from build123d import *

# Parameters (mm, degrees)
SKETCH1_R           = 1.8288
BOSS_EXTRUDE1_DEPTH = 3.175
SKETCH2_R           = 1.63195
SKETCH2_R_2         = 5.715
SKETCH2_R_3         = 1.524
CUT_EXTRUDE1_DEPTH  = 4.175
SKETCH3_R           = 1.375
CUT_EXTRUDE2_DEPTH  = 4.175


with BuildPart() as part:
    # Sketch1 → Boss-Extrude1 (new body)
    with BuildSketch(Plane(origin=(0, 0, 0), x_dir=(1, 0, 0), z_dir=(0, 1, 0))):
        Polygon((-226.6315, 82.55), (-194.8815, 82.55), (-194.8815, 69.85), (-188.5315, 69.85), (-188.5315, 82.55), (-38.1, 82.55), (-38.1, 69.85), (-31.75, 69.85), (-31.75, 82.55), (0, 82.55), (0, 51.435), (-3.175, 51.435), (-3.175, 31.115), (0, 31.115), (0, 0), (-31.75, 0), (-31.75, 12.7), (-38.1, 12.7), (-38.1, 0), (-188.5315, 0), (-188.5315, 12.7), (-194.8815, 12.7), (-194.8815, 0), (-226.6315, 0), (-226.6315, 31.115), (-223.4565, 31.115), (-223.4565, 51.435), (-226.6315, 51.435), align=None)
        with Locations((-113.31575, 41.275)):
            Circle(SKETCH1_R, mode=Mode.SUBTRACT)
    extrude(amount=BOSS_EXTRUDE1_DEPTH)

    # Sketch2 → Cut-Extrude1 (cut, through all)
    with BuildSketch(Plane(origin=(0, 3.175, 0), x_dir=(1, 0, 0), z_dir=(0, 1, 0))):
        with Locations((-87.63, 27.305)):
            Circle(SKETCH2_R)
        with Locations((-69.85, 27.305)):
            Circle(SKETCH2_R)
        with Locations((-69.85, 55.245)):
            Circle(SKETCH2_R)
        with Locations((-87.63, 55.245)):
            Circle(SKETCH2_R)
        with Locations((-78.74, 41.275)):
            Circle(SKETCH2_R_2)
        with Locations((-129.82575, 41.275)):
            Circle(SKETCH2_R_3)
        with Locations((-96.80575, 41.275)):
            Circle(SKETCH2_R_3)
    extrude(amount=-CUT_EXTRUDE1_DEPTH, mode=Mode.SUBTRACT)

    # Sketch3 → Cut-Extrude2 (cut, through all)
    with BuildSketch(Plane(origin=(0, 3.175, 0), x_dir=(1, 0, 0), z_dir=(0, 1, 0))):
        with Locations((-174.4315, 57.97)):
            Circle(SKETCH3_R)
        with Locations((-213.9315, 57.97)):
            Circle(SKETCH3_R)
        with Locations((-213.9315, 77.47)):
            Circle(SKETCH3_R)
        with Locations((-174.4315, 77.47)):
            Circle(SKETCH3_R)
    extrude(amount=-CUT_EXTRUDE2_DEPTH, mode=Mode.SUBTRACT)


solid = part.part
Input: part model. Units: mm. Frame: model coordinates. Give positions to 0.01 mm unless a question says otherwise; leave off trailing zeros. Answer as a JSON object with one key per item and string values. Group by question number.
Item 1: Pull-direction query (X, two-part tool) for faces 1 (the cylindrical face through (-113.55, 1.57, -43.09)), 2 (the flat face through (-112, 0, -51)); classes: released by +X, released by -X, zero draft, split by the parting line, or undercut.
Item 2: Cut plane A-A, the plane y = 1.4. State how many separate pieces and enclosed holes the cut face has, and give its area (3 significant figures).
Item 3: Line query: probe 1 along X at (y, z) = (0.55, -74); probe 2 along Z at (x, y) = (-69.85, 1.55); probe 3 along X at (y, z) = (1.2, -77.47). Output: solid intervals per line, ascending.
Item 4: Pin query (flat end, axial travel): P1, Ø5, axis at x = -107.5, z = -11, coming from the -Y side; P2, Ø1.6, axis at x = -190, y = 2, coming from the +Z side. Return the tip coordinate at first contact, or that it passes through.
Checks:
{
 "1": {"face 1": "undercut", "face 2": "zero draft"},
 "2": {"separate pieces": "1", "enclosed holes": "12", "area": "18,100 mm²"},
 "3": {"probe 1": "x = -226.63 to -194.88, -188.53 to -38.1, -31.75 to 0", "probe 2": "z = -82.55 to -56.88, -53.61 to -28.94, -25.67 to 0", "probe 3": "x = -226.63 to -215.31, -212.56 to -194.88, -188.53 to -175.81, -173.06 to -38.1, -31.75 to 0"},
 "4": {"P1": "stops at y = 0", "P2": "stops at z = -12.7"}
}
